from build123d import *

# Parameters (mm, degrees)
SKETCH_1_R          = 6
SKETCH_1_R_2        = 3
EXTRUDE_1_DEPTH     = 3.825
FILLET_1_R          = 0.1
SKETCH_2_R          = 1.5
CUT_EXTRUDE_1_DEPTH = 7.65


with BuildPart() as part:
    # 草圖1 → 填料-伸長1 (new, symmetric)
    with BuildSketch(Plane.XY):
        Circle(SKETCH_1_R)
        Circle(SKETCH_1_R_2, mode=Mode.SUBTRACT)
    extrude(amount=EXTRUDE_1_DEPTH, both=True)

    # 圓角1
    fillet_1_edges = [part.edges().sort_by_distance(p)[0] for p in [
        (-6, 0, 3.825),
        (-3, 0, -3.825),
        (-3, 0, 3.825),
    ]]
    fillet(fillet_1_edges, radius=FILLET_1_R)

    # 草圖2 → 除料-伸長1 (cut)
    with BuildSketch(Plane(origin=(0, 0, 0), x_dir=(1, 0, 0), z_dir=(0, 1, 0))):
        with Locations(Location((0, 0, 0), (0, 0, 90))):
            Circle(SKETCH_2_R)
    extrude(amount=CUT_EXTRUDE_1_DEPTH, mode=Mode.SUBTRACT)


solid = part.part
Could you check a few things on this model? Use its own coordinates, in mm. Give positions to 0.01 mm unless a question says otherwise; leave off trailing zeros. Order: outer loops, then holes, each group sorted by start corner. A loop starts at its lowest first (then second) coordinate and runs counter-clockwise, first axis right, second up. Notation, with made-up numbers: (19.5, 76.25) -> (45.5, 76.25) arc R18 ccw to (45.5, 80.25) -> close; hole circle Ø3 at (59.25, 15.5). An arc over 180 degrees is marked (long way). Answer in a Markdown table with one row per item. Add a question column.
Item 1: I'm going to push flat-ended pins straight in: P1, Ø5.5, axis at x = 0, y = 0, coming from the -Z side; P2, Ø4, axis at x = -3.5, z = -3, coming from the +Y side. Where does each tip first touch, or does it pass through?
Item 2: We'd pull the mould along Z, two halves only. Please class faces 1 (the flat face through (3, -3, -3.825)), 2 (the cylindrical face through (-0.45, 4.28, -1.43)), 3 (the flat face through (3, -3, 3.825)): pulls with the +Z half, pulls with the -Z half, needs draft (parallel to the pull), parting line crosses it, or undercut.
Item 3: Imagine slicing it at A-A (y = 0). List the corners of the cut face in (x, z) for me (3 decimals).
Item 4: Imagine slicing it at D-D (z = 1). List the corners of the cut face in (x, y) for me, and give its area (3 significant figures).
Item 5: Please list where these lines run through material, in increasing order: probe 1 along X at (y, z) = (3.95, 0); probe 2 along Y at (x, z) = (-0.25, 2.5); probe 3 along X at (y, z) = (3.5, 0).
Item 6: Imagine slicing it at B-B (x = 0). List the corners of the cut face in (y, z) for me (3 decimals).
Item 7: Imagine slicing it at C-C (z = 2.75). List the corners of the cut face in (x, y) for me, and give its area (3 significant figures).
Result:
| question | item | result |
|---|---|---|
| 1 | P1 | through |
| 1 | P2 | y = 5.81 |
| 2 | face 1 | pulls with the -Z half |
| 2 | face 2 | undercut |
| 2 | face 3 | pulls with the +Z half |
| 3 | outline | (-6, -3.825) -> (-3.1, -3.825) arc R0.1 ccw to (-3, -3.725) -> (-3, 3.725) arc R0.1 ccw to (-3.1, 3.825) -> (-5.9, 3.825) arc R0.1 ccw to (-6, 3.725) -> close; (3, -3.725) arc R0.1 ccw to (3.1, -3.825) -> (6, -3.825) -> (6, 3.725) arc R0.1 ccw to (5.9, 3.825) -> (3.1, 3.825) arc R0.1 ccw to (3, 3.725) -> close |
| 4 | outline | (-1.12, 2.78) -> (-1.12, 5.89) arc R6 ccw (long way) to (1.12, 5.89) -> (1.12, 2.78) arc R3 cw (long way) to start |
| 4 | area | 78.0 mm2 |
| 5 | probe 1 | -4.52 to -1.5, 1.5 to 4.52 |
| 5 | probe 2 | -5.99 to -2.99, 2.99 to 5.99 |
| 5 | probe 3 | -4.87 to -1.5, 1.5 to 4.87 |
| 6 | outline | (-6, -3.825) -> (-3.1, -3.825) arc R0.1 ccw to (-3, -3.725) -> (-3, 3.725) arc R0.1 ccw to (-3.1, 3.825) -> (-5.9, 3.825) arc R0.1 ccw to (-6, 3.725) -> close; (3, -3.725) arc R0.1 ccw to (3.1, -3.825) -> (6, -3.825) -> (6, -1.5) -> (3, -1.5) -> close; (3, 1.5) -> (6, 1.5) -> (6, 3.725) arc R0.1 ccw to (5.9, 3.825) -> (3.1, 3.825) arc R0.1 ccw to (3, 3.725) -> close |
| 7 | outline | circle Ø12 at (0, 0); hole circle Ø6 at (0, 0) |
| 7 | area | 84.8 mm2 |
